Model file for the job. Use its own axes, mm. Face numbers are marked on the shaded views. Round coordinates to 2 decimals unless told otherwise and drop trailing zeros. Order: outer loops, then holes, each group sorted by start corner. A loop starts at its lowest first (then second) coordinate and runs counter-clockwise, first axis right, second up. Notation, with made-up numbers: (12.25, -35.75) - (36.25, -35.75) arc R21 ccw to (36.25, 1.25) - close; hole circle Ø4 at (-17.75, -35). An arc over 180 degrees is marked (long way). Put each result on its own line as item: value. Start each with the question number.
Item 1: Pin check, flat tips, straight feed: pin 1 Ø1 at (x, y) = (99, -2) entering from -Z; pin 2 Ø2 at (x, z) = (51, 0) entering from +Y. Stop position of each tip, or through.
Item 2: Mould opens along Z. For the marked faces 1, 2, 3 and 4 say: pulls with the +Z half, pulls with the -Z half, needs draft (parallel to the pull), parting line crosses it, or undercut.
Item 3: Probe probe 1 along Y at (x, z) = (108, 103.5); probe 2 along Y at (x, z) = (94, -108); probe 3 along Y at (x, z) = (51, 94.5). List the from-to ranges inside material, lowest first.
Item 4: Saw through at A-A on z = 53. List the corners of the cut face in (x, y).
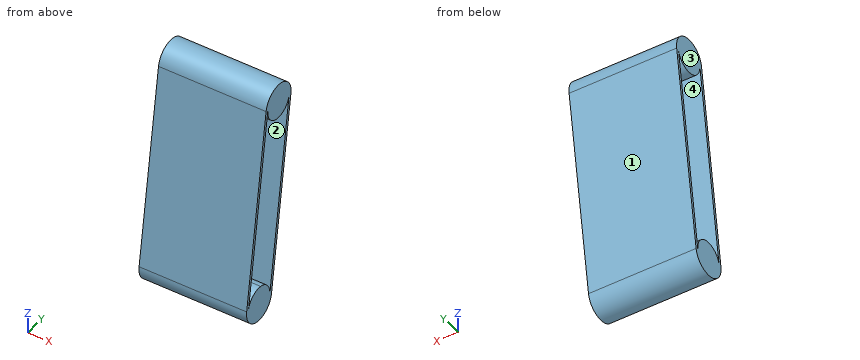
Autodesk Inventor part; units mm, degrees
ref_plane "YZ Plane" through (0, 0, 0) normal (1, 0, 0) x (0, 1, 0)
ref_plane "XZ Plane" through (0, 0, 0) normal (0, 1, 0) x (-1, 0, 0)
ref_plane "XY Plane" through (0, 0, 0) normal (0, 0, 1) x (1, 0, 0)
sketch "Sketch3" plane through (0, 0, 0) normal (1, 0, 0) x (0, 1, 0)
  line L0 (17.2137, 115.1798) -> (-17.2137, -115.1798) construction
  line L1 (-4.7671, 118.4649) -> (-39.1946, -111.8947)
  line L2 (4.7671, -118.4649) -> (39.1946, 111.8947)
  arc A0 (39.1946, 111.8947) -> (-4.7671, 118.4649) centre (17.2137, 115.1798) ccw
  arc A1 (-39.1946, -111.8947) -> (4.7671, -118.4649) centre (-17.2137, -115.1798) ccw
  line L3 (0, 0) -> (232.918, 0) construction
  line L4 (36.0545, 112.364) -> (1.627, -117.9956)
  arc A2 (-36.0545, -112.364) -> (1.627, -117.9956) centre (-17.2137, -115.1798) ccw
  line L5 (-36.0545, -112.364) -> (-1.627, 117.9956)
  arc A3 (36.0545, 112.364) -> (-1.627, 117.9956) centre (17.2137, 115.1798) ccw
  ellipse E0 centre (17.2137, 115.1798) end of major axis (36.0545, 112.364) minor radius 19.05
  ellipse E1 centre (-17.2137, -115.1798) end of major axis (1.627, -117.9956) minor radius 19.05
  point P0 (-36.0545, -112.364)
  dimension "d8" = 116.459
  dimension "d9" = 98.5
  dimension "d10" = 44.45
  dimension "d11" = 3.175
extrude "Extrusion3" add sketch "Sketch3" along normal blind 127 contours A0 L2 A1 L1 | E0 A3 | A2 E1
properties part number "ShootingMech_Housing4"
Results found:
1. pin 1: stops at z = -131.84
1. pin 2: stops at y = 22.62
2. face 1: pulls with the -Z half
2. face 2: undercut
2. face 3: needs draft
2. face 4: undercut
3. probe 1: y = -7 to -3.79, 2.16 to 32.26, 34.73 to 37.94
3. probe 2: y = -38.61 to -35.4, -34.86 to 0.43, 3.12 to 6.33
3. probe 3: y = -8.35 to -5.14, 33.38 to 36.59
4. outline: (0, -14.55) - (127, -14.55) - (127, -11.34) - (0, -11.34) - close; (0, 27.18) - (127, 27.18) - (127, 30.39) - (0, 30.39) - close
